Model file for the job. Use its own axes, mm. Face numbers are marked on the shaded views. A direction names the side the tool comes from. Round coordinates to 2 decimals unless told otherwise and drop trailing zeros. Order: outer loops, then holes, each group sorted by start corner. A loop starts at its lowest first (then second) coordinate and runs counter-clockwise, first axis right, second up. Notation, with made-up numbers: (-39, 11) -> (8, 11) arc R19 ccw to (8, 43) -> close; hole circle Ø1 at (15.5, 19.5). An arc over 180 degrees is marked (long way). Put each result on its own line as item: value. Start each with the question number.
Q1. 3-axis set-ups, long thin cutter, end or side, ignore diameter. For the marked faces 1, 2 and 3: which of +Z, -Z, +X, -X, +Y, -Y reach the whole face in a straight line?
Q2. Probe L1, parallel to Y at x = 81, z = 0; L2, parallel to Z at x = 52, y = 0. List the from-to ranges inside material, lowest first.
Q3. Pull direction Y, two halves, no side cores. Call the marked faces 4 and 5: released by +Y, released by -Y, zero draft, split by the parting line, or undercut.
Q4. Cut at D-D, the plane x = 169. List the corners of the cut face in (y, z), and give its area (3 significant figures).
Q5. Flat gauge pins, fed straight in: P1, Ø1, axis at x = 73.5, z = 27.5, coming from the -Y side; P2, Ø5, axis at y = 5, z = 30, coming from the +X side; P3, Ø1.5, axis at y = -25.5, z = 23, coming from the +X side; P4, Ø24, axis at y = -11, z = 9, coming from the -X side. Where does each tip first touch, or does it go through?
Q6. Cut at C-C, the plane x = 125.5. List the corners of the cut face in (y, z).
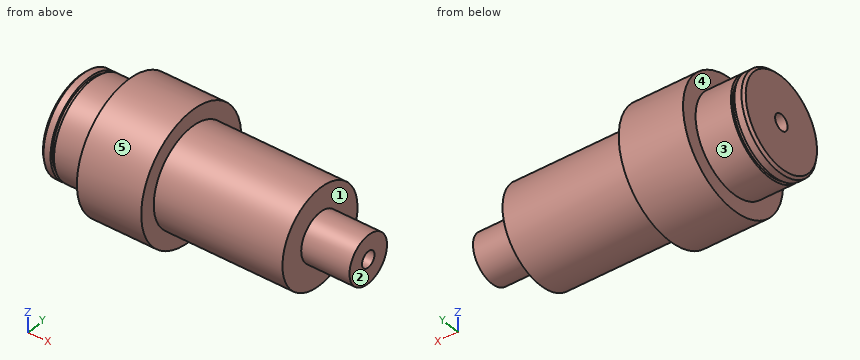
from build123d import *

# Parameters (mm, degrees)
F2_SIZE = 1.5


with BuildPart() as f1:
    # F0 (on Front) → F1 (revolve)
    with BuildSketch(Plane.XZ):
        Polygon((5.85, 30), (0, 30), (0, 5), (180, 5), (180, 15), (150, 15), (150, 30), (70, 30), (70, 40), (30, 40), (30, 30), (8, 30), (8, 28.5), (5.85, 28.5), align=None)
    revolve(axis=Axis((74.107222, 0, 0), (1, 0, 0)))

    # F2
    f2_edges = [f1.edges().sort_by_distance(p)[0] for p in [
        (0, 0, -30),
    ]]
    chamfer(f2_edges, length=F2_SIZE)


solid = f1.part
Ans:
1. face 1: +X
1. face 2: +Z, -Z, +X, +Y, -Y
1. face 3: -X
2. L1: y = -30 to -5, 5 to 30
2. L2: z = -40 to -5, 5 to 40
3. face 4: zero draft
3. face 5: split by the parting line
4. outline: circle Ø30 at (0, 0); hole circle Ø10 at (0, 0)
4. area: 628 mm^2
5. P1: stops at y = -13.08
5. P2: stops at x = 150
5. P3: stops at x = 70
5. P4: stops at x = 0
6. outline: circle Ø60 at (0, 0); hole circle Ø10 at (0, 0)
